Here's how the part is built. I have some questions about the finished solid (model axes, mm). Face numbers are marked on the shaded views. Round coordinates to 2 decimals unless told otherwise and drop trailing zeros. Loops run counter-clockwise (first coordinate to the right, second up) from the corner with the lowest first, then second, coordinate; pieces in that order, holes last. Notation, with made-up numbers: (62, 68) - (69, 68) arc R37 ccw to (69, 105) - close; hole circle Ø11 at (81, 76.25). An arc over 180 degrees is marked (long way). Answer as a JSON object with one key per item and string values. Group by question number.
1) If we mould it in two halves opening along Y, with no side actions, what happens to the marked faces 1, 2 and 3? For each: pulls with the +Y half, pulls with the -Y half, needs draft (parallel to the pull), parting line crosses it, or undercut.
2) I want a section at A-A, the plane x = 89.5. Please give me the cut outline in (y, z), then the cut area to 3 significant figures.
3) Will these pins go through, and if not, where does the flat tip stop? P1, Ø5, axis at x = 149.5, y = 4, coming from the +Z side; P2, Ø1.8, axis at x = 161, y = 4.5, coming from the +Z side.
4) If I drill on line 1 along Y through (x, z) = (59.5, 3); line 2 along Z through (x, y) = (54.5, 6.75); line 3 along Z through (x, y) = (152, 7), over which ranges is the centre line in solid material (lowest first)? Write a range as [from, to].
5) I want a section at B-B, the plane x = 149.5. Please give me the cut outline in (y, z), then the cut area to 4 significant figures.
Autodesk Inventor part; units mm, degrees
ref_plane "YZ Plane" through (0, 0, 0) normal (1, 0, 0) x (0, 1, 0)
ref_plane "XZ Plane" through (0, 0, 0) normal (0, 1, 0) x (-1, 0, 0)
ref_plane "XY Plane" through (0, 0, 0) normal (0, 0, 1) x (1, 0, 0)
sketch "Sketch1" plane through (0, 0, 0) normal (0, 0, 1) x (1, 0, 0)
  line L0 (0, 0) -> (167, 0)
  line L1 (167, 0) -> (167, 10)
  line L2 (167, 10) -> (0, 10)
  line L3 (0, 10) -> (0, 0)
  circle A0 centre (59.5, 5) radius 1.6
  circle A1 centre (101.5, 5) radius 1.6
  circle A2 centre (162, 5) radius 1.6
  circle A3 centre (149.5, 5) radius 1.6
  circle A4 centre (15, 5) radius 1.6
  circle A5 centre (5, 5) radius 1.6
  dimension "d1" = 10
  dimension "d2" = 90
  dimension "d4" = 3.2
  dimension "d6" = 3.2
  dimension "d7" = 3.2
  dimension "d8" = 42
  dimension "d9" = 60.5
  dimension "d26" = 3.2
  dimension "d27" = 48
  dimension "d28" = 3.2
  dimension "d29" = 44.5
  dimension "d32" = 15
  dimension "d33" = 5
  dimension "d61" = 3.2
  dimension "d62" = 10
  dimension "d63" = 12.5
ref_plane "Work Plane2" through (0, 0, 0) normal (0, -1, 0) x (1, 0, 0)
sketch "Sketch2" plane through (0, 0, 0) normal (0, -1, 0) x (1, 0, 0)
  circle A0 centre (54.5, 7) radius 1.6
  circle A1 centre (124.5, 7) radius 1.6
  circle A2 centre (89.5, 7) radius 1.6
  point P0 (0, 0)
  dimension "d13" = 3.2
  dimension "d15" = 3.2
  dimension "d16" = 70
  dimension "d17" = 3.2
  dimension "d18" = 35
  dimension "d64" = 54.5
  dimension "d65" = 35
ref_plane "Work Plane1" through (0, 0, 11) normal (0, 0, 1) x (1, 0, 0)
extrude "klocek" add sketch "Sketch1" along normal blind 11
ref_plane "Work Plane3" through (0, 0, 0) normal (0, -1, 0) x (1, 0, 0)
extrude "prowadzenie osi" cut sketch "Sketch2" against normal up to next
ref_plane "Work Plane4" through (0, 0, 0) normal (0, -1, 0) x (1, 0, 0)
sketch "Sketch7" plane through (0, 0, 0) normal (0, -1, 0) x (1, 0, 0)
  line L0 (0, 11) -> (0, 0)
  line L1 (0, 11) -> (167, 11)
  line L2 (0, 11) -> (40, 11)
  line L3 (40, 11) -> (0, 0)
  point P0 (0, -1.8333)
  dimension "d86" = 11
  dimension "d87" = 40
sketch "Sketch8" plane through (0, 0, 0) normal (0, -1, 0) x (1, 0, 0)
  line L0 (167, 0) -> (167, 11)
  line L1 (167, 11) -> (167, 5)
  line L2 (167, 11) -> (0, 11)
  line L3 (167, 11) -> (137, 11)
  line L4 (137, 11) -> (167, 5)
  point P0 (0, 0)
  point P1 (40.8333, 11)
  dimension "d80" = 6
  dimension "d81" = 30
extrude "przedni skos" cut sketch "Sketch7" against normal up to next
extrude "tylni skos" cut sketch "Sketch8" against normal up to next
ref_plane "Work Plane7" through (0, 0, 11) normal (0, 0, 1) x (1, 0, 0)
sketch "Sketch5" plane through (0, 0, 11) normal (0, 0, 1) x (1, 0, 0)
  line L0 (62.9064, 5) -> (61.2032, 2.05)
  line L1 (61.2032, 2.05) -> (57.7968, 2.05)
  line L2 (57.7968, 2.05) -> (56.0936, 5)
  line L3 (56.0936, 5) -> (57.7968, 7.95)
  line L4 (57.7968, 7.95) -> (61.2032, 7.95)
  line L5 (61.2032, 7.95) -> (62.9064, 5)
  circle A0 centre (101.5, 5) radius 1.6
  line L6 (98.0936, 5) -> (99.7968, 7.95)
  line L7 (99.7968, 7.95) -> (103.2032, 7.95)
  line L8 (103.2032, 7.95) -> (104.9064, 5)
  line L9 (104.9064, 5) -> (103.2032, 2.05)
  line L10 (103.2032, 2.05) -> (99.7968, 2.05)
  line L11 (99.7968, 2.05) -> (98.0936, 5)
  point P0 (59.5, 5)
  point P1 (119.5, 5)
  dimension "d45" = 5.9
  dimension "d98" = 5.9
extrude "hex insert middle" cut sketch "Sketch5" against normal blind 3
ref_plane "Work Plane6" through (0, 0, 11) normal (0, 0, 1) x (1, 0, 0)
sketch "Sketch9" plane through (0, 0, 11) normal (0, 0, 1) x (1, 0, 0)
  circle A0 centre (149.5, 5) radius 1.6
  line L0 (152.9064, 5) -> (151.2032, 2.05)
  line L1 (151.2032, 2.05) -> (147.7968, 2.05)
  line L2 (147.7968, 2.05) -> (146.0936, 5)
  line L3 (146.0936, 5) -> (147.7968, 7.95)
  line L4 (147.7968, 7.95) -> (151.2032, 7.95)
  line L5 (151.2032, 7.95) -> (152.9064, 5)
  point P0 (0, 0)
  point P1 (153, 5)
  dimension "d99" = 5.9
extrude "hex insert rear 1" cut sketch "Sketch9" against normal blind 6
ref_plane "Work Plane5" through (0, 0, 11) normal (0, 0, 1) x (1, 0, 0)
sketch "Sketch10" plane through (0, 0, 11) normal (0, 0, 1) x (1, 0, 0)
  line L0 (160.2968, 7.95) -> (163.7032, 7.95)
  line L1 (163.7032, 7.95) -> (165.4064, 5)
  line L2 (165.4064, 5) -> (163.7032, 2.05)
  line L3 (163.7032, 2.05) -> (160.2968, 2.05)
  line L4 (160.2968, 2.05) -> (158.5936, 5)
  line L5 (158.5936, 5) -> (160.2968, 7.95)
  point P0 (0, 0)
  point P1 (162, 5)
  point P2 (162, 5)
  dimension "d72" = 5.9
extrude "hex insert rear 2" cut sketch "Sketch10" against normal blind 7.5
sketch "Sketch13" plane through (0, 0, 11) normal (0, 0, 1) x (1, 0, 0)
  circle A0 centre (5, 5) radius 1.6
  line L0 (8.4064, 5) -> (6.7032, 2.05)
  line L1 (6.7032, 2.05) -> (3.2968, 2.05)
  line L2 (3.2968, 2.05) -> (1.5936, 5)
  line L3 (1.5936, 5) -> (3.2968, 7.95)
  line L4 (3.2968, 7.95) -> (6.7032, 7.95)
  line L5 (6.7032, 7.95) -> (8.4064, 5)
  point P0 (0, 0)
  dimension "d90" = 5.9
extrude "hex insert front 1" cut sketch "Sketch13" against normal through all
sketch "Sketch16" plane through (0, 0, 11) normal (0, 0, 1) x (1, 0, 0)
  circle A0 centre (15, 5) radius 1.6
  line L0 (18.4064, 5) -> (16.7032, 2.05)
  line L1 (16.7032, 2.05) -> (13.2968, 2.05)
  line L2 (13.2968, 2.05) -> (11.5936, 5)
  line L3 (11.5936, 5) -> (13.2968, 7.95)
  line L4 (13.2968, 7.95) -> (16.7032, 7.95)
  line L5 (16.7032, 7.95) -> (18.4064, 5)
  point P0 (0, 0)
  dimension "d93" = 5.9
extrude "hex insert front 2" cut sketch "Sketch16" against normal blind 9
sketch "Sketch17" plane through (0, 0, 0) normal (0, 0, -1) x (-1, 0, 0)
  line L0 (0, 10) -> (0, 0)
  line L1 (0, 0) -> (-3.2968, 0)
  line L2 (-3.2968, 0) -> (-3.2968, 10.0042)
  line L3 (-3.2968, 10.0042) -> (0, 10.0042)
  line L4 (0, 10.0042) -> (0, 0)
extrude "Extrusion20" cut sketch "Sketch17" against normal up to next
properties part number "wheel_support_extra_short"
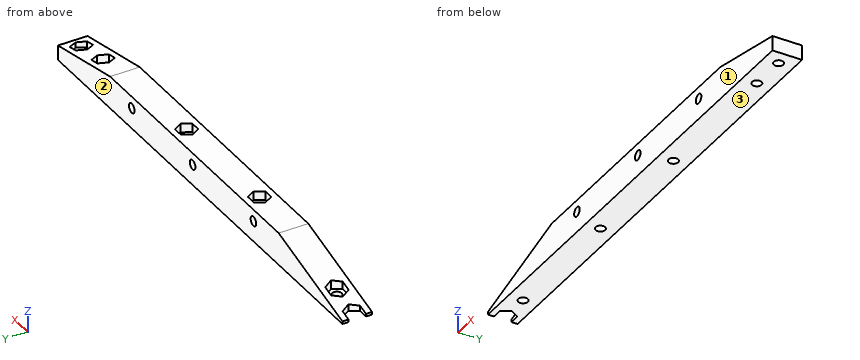
Outcome:
{
 "1": {"face 1": "pulls with the -Y half", "face 2": "pulls with the +Y half", "face 3": "needs draft"},
 "2": {"outline": "(0, 0) - (10, 0) - (10, 5.4) - (0, 5.4) - close; (0, 8.6) - (10, 8.6) - (10, 11) - (0, 11) - close", "area": "78.0 mm^2"},
 "3": {"P1": "z = 8.97", "P2": "z = 3.5"},
 "4": {"line 1": "[0, 3.4], [6.6, 10]", "line 2": "[0, 5.4], [8.6, 11]", "line 3": "[0, 8]"},
 "5": {"outline": "(0, 0) - (3.4, 0) - (3.4, 5) - (2.05, 5) - (2.05, 8.5) - (0, 8.5) - close; (6.6, 0) - (10, 0) - (10, 8.5) - (7.95, 8.5) - (7.95, 5) - (6.6, 5) - close", "area": "48.35 mm^2"}
}
